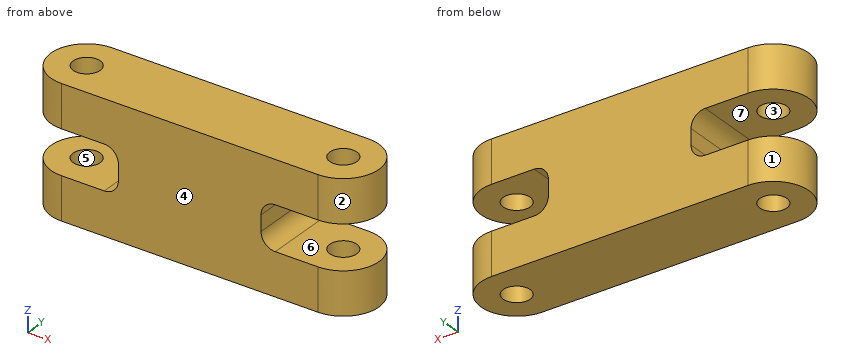
```python
from build123d import *

# Parameters (mm, degrees)
EXTRUDE_START       = -9.1
EXTRUDE_1_DEPTH     = 6
SKETCH_5_R          = 1.9
CUT_EXTRUDE_5_DEPTH = 42.737273509
SKETCH_6_R          = 1.9
CUT_EXTRUDE_6_DEPTH = 10
SKETCH_7_W          = 20
SKETCH_7_H          = 10
EXTRUDE_2_DEPTH     = 3.1
FILLET_1_R          = 2


with BuildPart() as part:
    # ｽｹｯﾁ1 → ﾎﾞｽ - 押し出し1 (new body)
    with BuildSketch(Plane.XY.offset(EXTRUDE_START)):
        with BuildLine():
            Line((0, 5), (-36, 5))
            ThreePointArc((-36, 5), (-41, 0), (-36, -5))
            Line((-36, -5), (0, -5))
            ThreePointArc((0, -5), (5, 0), (0, 5))
        make_face()
    extrude_1 = extrude(amount=EXTRUDE_1_DEPTH)

    # ｽｹｯﾁ5 → ｶｯﾄ - 押し出し5 (cut, through all)
    with BuildSketch(Plane.XY.offset(-3.1)):
        with Locations((-36, 0)):
            Circle(SKETCH_5_R)
    cut_extrude_5 = extrude(amount=-CUT_EXTRUDE_5_DEPTH, mode=Mode.SUBTRACT)

    # ｽｹｯﾁ6 → ｶｯﾄ - 押し出し6 (cut)
    with BuildSketch(Plane.XY.offset(-3.1)):
        Circle(SKETCH_6_R)
    cut_extrude_6 = extrude(amount=-CUT_EXTRUDE_6_DEPTH, mode=Mode.SUBTRACT)

    # ｽｹｯﾁ7 → ﾎﾞｽ - 押し出し2 (add)
    with BuildSketch(Plane.XY.offset(-3.1)):
        with Locations((-18, 0)):
            Rectangle(SKETCH_7_W, SKETCH_7_H)
    extrude_2 = extrude(amount=EXTRUDE_2_DEPTH)

    # ﾐﾗｰ3: ﾎﾞｽ - 押し出し1, ｶｯﾄ - 押し出し5, ｶｯﾄ - 押し出し6, ﾎﾞｽ - 押し出し2 across plane
    add(extrude_1.mirror(Plane.XY))
    add(cut_extrude_5.mirror(Plane.XY), mode=Mode.SUBTRACT)
    add(cut_extrude_6.mirror(Plane.XY), mode=Mode.SUBTRACT)
    add(extrude_2.mirror(Plane.XY))

    # ﾌｨﾚｯﾄ1
    fillet_1_edges = [part.edges().sort_by_distance(p)[0] for p in [
        (-8, 0, -3.1),
        (-28, 0, -3.1),
        (-8, 0, 3.1),
        (-28, 0, 3.1),
    ]]
    fillet(fillet_1_edges, radius=FILLET_1_R)


solid = part.part
```
Build history of the part. All positions in model axes, mm. Face numbers are marked on the shaded views. A direction names the side the tool comes from. Round coordinates to 2 decimals unless told otherwise and drop trailing zeros. Write each loop counter-clockwise with the first axis right and the second up, starting at its lowest first coordinate (ties: lowest second). Pieces come first, ordered by that corner, then holes. Notation, with made-up numbers: (62, -29.75) -> (118, -29.75) arc R25 ccw to (118, -1.75) -> close; hole circle Ø3 at (-33.75, -24.5). An arc over 180 degrees is marked (long way). Put each result on its own line as item: value.
Item 1: Flat gauge pins, fed straight in: P1, Ø5, axis at x = -36, y = 0, coming from the +Z side; P2, Ø2.5, axis at y = -1, z = -0.5, coming from the -X side; P3, Ø3, axis at x = -36, y = 0, coming from the +Z side; P4, Ø1.5, axis at y = 1, z = -6.5, coming from the -X side. Where does each tip first touch, or does it go through?
Here are the results:
P1: stops at z = 9.1
P2: stops at x = -28.11
P3: passes through
P4: stops at x = -40.99
Item 2: Tool access for the marked faces 5, 6 and 7: list every direction of +Z, -Z, +X, -X, +Y, -Y with a clear straight run to the whole face (end or side of a thin tool).
Here are the results:
face 5: +Z, -Z
face 6: +X, +Y, -Y
face 7: -X, +Y, -Y
Item 3: Slice it at A-A, the plane y = 0. Count the separate pieces of the cut face and the enclosed holes in it, plus the area to 3 significant figures.
Here are the results:
separate pieces: 5
enclosed holes: 0
area: 588 mm^2
Item 4: Slice it at C-C, the plane z = -2.5. Give the cut face in (x, y).
Here are the results:
outline: (-28.57, -5) -> (-7.43, -5) -> (-7.43, 5) -> (-28.57, 5) -> close
Item 5: Slice it at B-B, the plane y = 3. Give the cut face in (x, z), plus the area to 3 significant figures.
Here are the results:
outline: (-40, -9.1) -> (4, -9.1) -> (4, -3.1) -> (-6, -3.1) arc R2 cw to (-8, -1.1) -> (-8, 1.1) arc R2 cw to (-6, 3.1) -> (4, 3.1) -> (4, 9.1) -> (-40, 9.1) -> (-40, 3.1) -> (-30, 3.1) arc R2 cw to (-28, 1.1) -> (-28, -1.1) arc R2 cw to (-30, -3.1) -> (-40, -3.1) -> close
area: 655 mm^2
Item 6: Wall check: probe 1 along X at (y, z) = (0, 4.85); probe 2 along Z at (x, y) = (-34, 1.25); probe 3 along Y at (x, z) = (-36, 4.3). Give the ranges that are in metal, low to high. Write a range as from..to.
Here are the results:
probe 1: x = -41..-37.9, -34.1..-1.9, 1.9..5
probe 2: z = -9.1..-3.1, 3.1..9.1
probe 3: y = -5..-1.9, 1.9..5
Item 7: Two-plate mould, pull along X, no slides. Class the marked faces 1, 2, 3 and 4: pulls with the +X half, pulls with the -X half, needs draft (parallel to the pull), parting line crosses it, or undercut.
Here are the results:
face 1: pulls with the -X half
face 2: pulls with the +X half
face 3: undercut
face 4: needs draft
